Geometry check sheet. Reference: the model listing, model coordinates, mm. A direction names the side the tool comes from. Round coordinates to 2 decimals unless told otherwise and drop trailing zeros. Order: outer loops, then holes, each group sorted by start corner. A loop starts at its lowest first (then second) coordinate and runs counter-clockwise, first axis right, second up. Notation, with made-up numbers: (-25.75, 53) - (-8.75, 53) arc R16 cw to (-8.75, 58) - close; hole circle Ø9 at (73.5, 80). An arc over 180 degrees is marked (long way). Write each question's results on one line, items separated by ' | '.
```python
from build123d import *

# Parameters (mm, degrees)
SKETCH3_W               = 19.05
SKETCH3_H               = 215.9
BOSS_EXTRUDE1_DEPTH     = 50.8
SKETCH5_W               = 254
SKETCH5_H               = 19.05
BOSS_EXTRUDE2_DEPTH     = 50.8
SKETCH6_W               = 12.7
SKETCH6_H               = 12.7
BOSS_EXTRUDE3_DEPTH     = 48.26
MIRROR3_COPY_1_SKETCH_W = 19.05
MIRROR3_COPY_1_SKETCH_H = 215.9
MIRROR3_COPY_1_DEPTH    = 50.8
MIRROR3_COPY_2_SKETCH_W = 12.7
MIRROR3_COPY_2_SKETCH_H = 12.7
MIRROR3_COPY_2_DEPTH    = 48.26
MIRROR3_COPY_3_SKETCH_W = 19.05
MIRROR3_COPY_3_SKETCH_H = 215.9
MIRROR3_COPY_3_DEPTH    = 50.8


with BuildPart() as part:
    # Sketch3 → Boss-Extrude1 (new body)
    with BuildSketch(Plane(origin=(0, 0, 0), x_dir=(1, 0, 0), z_dir=(0, 1, 0))):
        with Locations((-117.475, 0)):
            Rectangle(SKETCH3_W, SKETCH3_H)
    boss_extrude1 = extrude(amount=BOSS_EXTRUDE1_DEPTH)

    # Sketch5 → Boss-Extrude2 (add)
    with BuildSketch(Plane(origin=(0, 0, 0), x_dir=(1, 0, 0), z_dir=(0, 1, 0))):
        with Locations((0, -117.475)):
            Rectangle(SKETCH5_W, SKETCH5_H)
    boss_extrude2 = extrude(amount=BOSS_EXTRUDE2_DEPTH)

    # Sketch6 → Boss-Extrude3 (add)
    with BuildSketch(Plane(origin=(0, 0, 0), x_dir=(1, 0, 0), z_dir=(0, 1, 0))):
        with Locations((-101.6, -101.6)):
            Rectangle(SKETCH6_W, SKETCH6_H)
    boss_extrude3 = extrude(amount=BOSS_EXTRUDE3_DEPTH)

    # Mirror2: Boss-Extrude1, Boss-Extrude3 across plane
    add(boss_extrude1.mirror(Plane(origin=(0, 0, 0), x_dir=(0, 0, 1), z_dir=(1, 0, 0))))
    add(boss_extrude3.mirror(Plane(origin=(0, 0, 0), x_dir=(0, 0, 1), z_dir=(1, 0, 0))))

    # Mirror3: Boss-Extrude3, Boss-Extrude2 across plane
    add(boss_extrude3.mirror(Plane.XY))
    add(boss_extrude2.mirror(Plane.XY))

    # Mirror3 copy 1 sketch → Mirror3 copy 1 (add)
    with BuildSketch(Plane(origin=(0, 0, 0), x_dir=(-1, 0, 0), z_dir=(0, 1, 0))):
        with Locations((-117.475, 0)):
            Rectangle(MIRROR3_COPY_1_SKETCH_W, MIRROR3_COPY_1_SKETCH_H)
    extrude(amount=MIRROR3_COPY_1_DEPTH)

    # Mirror3 copy 2 sketch → Mirror3 copy 2 (add)
    with BuildSketch(Plane(origin=(0, 0, 0), x_dir=(-1, 0, 0), z_dir=(0, 1, 0))):
        with Locations((-101.6, -101.6)):
            Rectangle(MIRROR3_COPY_2_SKETCH_W, MIRROR3_COPY_2_SKETCH_H)
    extrude(amount=MIRROR3_COPY_2_DEPTH)

    # Mirror3 copy 3 sketch → Mirror3 copy 3 (add)
    with BuildSketch(Plane(origin=(0, 0, 0), x_dir=(1, 0, 0), z_dir=(0, 1, 0))):
        with Locations((-117.475, 0)):
            Rectangle(MIRROR3_COPY_3_SKETCH_W, MIRROR3_COPY_3_SKETCH_H)
    extrude(amount=MIRROR3_COPY_3_DEPTH)


solid = part.part
```
(1) Section check A-A (x = 99.5). Record the cut outline in (y, z), then the cut area to 3 significant figures.
Answers follow:
outline: (0, -127) - (50.8, -127) - (50.8, -107.95) - (48.26, -107.95) - (48.26, -95.25) - (0, -95.25) - close; (0, 95.25) - (48.26, 95.25) - (48.26, 107.95) - (50.8, 107.95) - (50.8, 127) - (0, 127) - close | area: 3,160 mm²
(2) Section check B-B (z = -74.5). Record the cut outline in (x, y).
Answers follow:
outline: (-127, 0) - (-107.95, 0) - (-107.95, 50.8) - (-127, 50.8) - close; (107.95, 0) - (127, 0) - (127, 50.8) - (107.95, 50.8) - close
(3) Material ranges on line 1 (Z direction, x = 45, y = 12.5); line 2 (Z direction, x = -105.5, y = 12.5), recorded low to high.
Answers follow:
line 1: -127 to -107.95, 107.95 to 127 | line 2: -127 to -95.25, 95.25 to 127
(4) Depth check by flat-ended pin: pin 1 Ø10 at (x, z) = (-102, -99) entering from +Y. Enter the tip coordinate at first touch or a pass-through.
Answers follow:
pin 1: y = 48.26
(5) Access from +Z, -Z, +X, -X, +Y, -Y to the whole of each face (thin tool, end or side, straight path). Record for faces 4 (the face through (-102, 48.26, -102)), 5 (the face through (95.25, 24, 102)), 6 (the face through (115, 0, 2)).
Answers follow:
face 4: +Y | face 5: +Y, -Y | face 6: +Z, -Z, +X, -X, -Y
(6) Draft check along Z on faces 1 (the face through (-127, 25, 2)), 2 (the face through (-2, 25, 127)), 3 (the face through (-102, 24, -95.25)). Enter one of: released by +Z, released by -Z, zero draft, split by the parting line, or undercut.
Answers follow:
face 1: zero draft | face 2: released by +Z | face 3: undercut
(7) Section check C-C (y = 29). Record the cut outline in (x, z).
Answers follow:
outline: (-127, -127) - (127, -127) - (127, 127) - (-127, 127) - close; hole (-107.95, -95.25) - (-95.25, -95.25) - (-95.25, -107.95) - (95.25, -107.95) - (95.25, -95.25) - (107.95, -95.25) - (107.95, 95.25) - (95.25, 95.25) - (95.25, 107.95) - (-95.25, 107.95) - (-95.25, 95.25) - (-107.95, 95.25) - close
(8) Section check D-D (x = 0.5). Record the cut outline in (y, z).
Answers follow:
outline: (0, -127) - (50.8, -127) - (50.8, -107.95) - (0, -107.95) - close; (0, 107.95) - (50.8, 107.95) - (50.8, 127) - (0, 127) - close
